Geometry check sheet. Reference: the model listing, model coordinates, mm. A direction names the side the tool comes from. Coordinates: 2 decimals unless noted, no trailing zeros. Write each loop counter-clockwise with the first axis right and the second up, starting at its lowest first coordinate (ties: lowest second). Pieces come first, ordered by that corner, then holes. Notation, with made-up numbers: (71, 48) - (117, 48) arc R14 ccw to (117, 52) - close; hole circle Ø10 at (-6, 13). An arc over 180 degrees is marked (long way). Answer as a JSON object with one key per item and string values. Group by question number.
from build123d import *

# Parameters (mm, degrees)
EXTRUDE_1_DEPTH = 16
SKETCH_2_W      = 24
SKETCH_2_H      = 148
CHAMFER_1_SIZE  = 5
CHAMFER_2_SIZE  = 2


with BuildPart() as part:
    # Эскиз1 → Бобышка-Вытянуть1 (new body)
    with BuildSketch(Plane.XZ.offset(164)):
        with BuildLine():
            Line((21.656407828, 30), (-21.656407828, 30))
            ThreePointArc((-21.656407828, 30), (-37, 0), (-21.656407828, -30))
            Line((-21.656407828, -30), (21.656407828, -30))
            ThreePointArc((21.656407828, -30), (37, 0), (21.656407828, 30))
        make_face()
    extrude(amount=-EXTRUDE_1_DEPTH)

    # Эскиз2 → Повернуть1 (revolve)
    with BuildSketch(Plane(origin=(0, 0, 0), x_dir=(-1, 0, 0), z_dir=(0, 0, -1)), mode=Mode.PRIVATE) as revolve_1_sk:
        with Locations((-12, -74)):
            Rectangle(SKETCH_2_W, SKETCH_2_H)
    revolve(revolve_1_sk.sketch.rotate(Axis((0, -148, 0), (0, 1, 0)), 270), axis=Axis((0, -148, 0), (0, 1, 0)))

    # Эскиз3 → Цековка для  болта с шестигранной головкой M301 (revolve, cut)
    with BuildSketch(Plane(origin=(0, 0, 0), x_dir=(0, 0, 1), z_dir=(1, 0, 0))):
        Polygon((0, 0), (0, 124.237604307), (16, 115), (16, 65), (11, 65), (11, 0), align=None)
    revolve(axis=Axis((0, 6.35, 0), (0, -1, 0)), mode=Mode.SUBTRACT)

    # Фаска1
    chamfer_1_edges = [part.edges().sort_by_distance(p)[0] for p in [
        (0, 0, -24),
        (-37, -164, 0),
        (37, -164, 0),
    ]]
    chamfer(chamfer_1_edges, length=CHAMFER_1_SIZE)

    # Фаска2
    chamfer_2_edges = [part.edges().sort_by_distance(p)[0] for p in [
        (0, 0, -11),
    ]]
    chamfer(chamfer_2_edges, length=CHAMFER_2_SIZE)


solid = part.part
(1) Draft check along X on faces 1 (the face through (-25, -148, 0)), 2 (the face through (-11, -65, 3)), 3 (the face through (7.21, -75.5, 22.89)). Enter one of: +X half, -X half, draft (parallel to the pull), parting line (faces both ways), or undercut.
(2) Section check B-B (y = -120.5). Record the cut outline in (x, z).
(3) Material ranges on L1, parallel to X at y = -39, z = 0; L2, parallel to X at y = -87, z = 0; L3, parallel to Y at x = -19.5, z = 15, recorded low to high. Write a range as [from, to].
(4) Gauge pin test, flat ends, axial feed: pin 1 (8 mm diameter, centred on x = -12.5, y = -26.5, fed in from -Z); pin 2 (1.5 mm diameter, centred on y = -71.5, z = 0, fed in from +X); pin 3 (6 mm diameter, centred on y = -109, z = 5.5, fed in from +X). Record the tip position at first contact, or that the pin passes through.
(5) Set-up check for faces 4 (the face through (2.713, -122.633, -0.602)), 5 (the face through (10.74, -33.06, -2.38)), 6 (the face through (37, -154, 0)): record each of +Z, -Z, +X, -X, +Y, -Y from which the full face is reachable in a straight line by a thin tool's end or side.
(6) Section check A-A (y = -19.5). Record the cut outline in (x, z), and give its area (3 significant figures).
Conclusion:
{
 "1": {"face 1": "draft", "face 2": "undercut", "face 3": "parting line"},
 "2": {"outline": "circle Ø48 at (0, 0); hole circle Ø12.95 at (0, 0)"},
 "3": {"L1": "x = [-24, -11], [11, 24]", "L2": "x = [-24, -16], [16, 24]", "L3": "y = [-164, -148]"},
 "4": {"pin 1": "stops at z = -22.44", "pin 2": "stops at x = 24", "pin 3": "stops at x = 23.87"},
 "5": {"face 4": "none", "face 5": "+Y", "face 6": "+X, +Y, -Y"},
 "6": {"outline": "circle Ø48 at (0, 0); hole circle Ø22 at (0, 0)", "area": "1,430 mm^2"}
}
